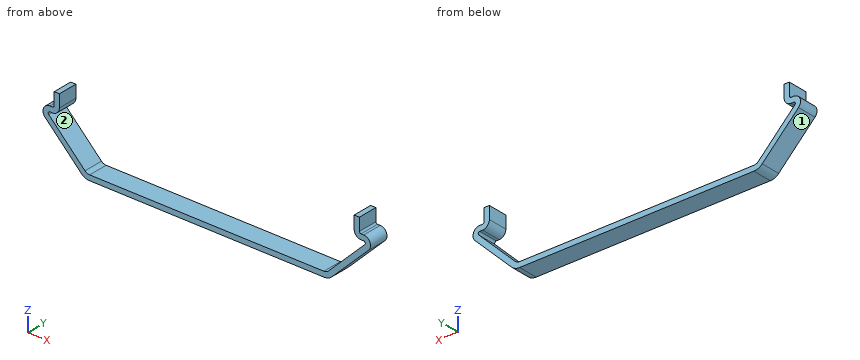
```python
from build123d import *

# Parameters (mm, degrees)
BOSS_EXTRUDE1_DEPTH = 1.5


with BuildPart() as part:
    # Sketch1 → Boss-Extrude1 (new, symmetric)
    with BuildSketch(Plane(origin=(0, 0, 0), x_dir=(1, 0, 0), z_dir=(0, 1, 0))):
        with BuildLine():
            Line((17.879536438, 11.70625), (-17.879536438, 11.70625))
            ThreePointArc((-17.879536438, 11.70625), (-18.26221987, 11.630129533), (-18.586643219, 11.413356781))
            Line((-18.586643219, 11.413356781), (-24.133026695, 5.866973305))
            ThreePointArc((-24.133026695, 5.866973305), (-24.187219883, 5.594525751), (-23.95625, 5.440196609))
            Line((-23.95625, 5.440196609), (-23.54375, 5.440196609))
            ThreePointArc((-23.54375, 5.440196609), (-22.805707297, 5.134489312), (-22.5, 4.396446609))
            Line((-22.5, 4.396446609), (-22.5, 2.5))
            Line((-22.5, 2.5), (-23.29375, 2.5))
            Line((-23.29375, 2.5), (-23.29375, 4.396446609))
            ThreePointArc((-23.29375, 4.396446609), (-23.366973305, 4.573223305), (-23.54375, 4.646446609))
            Line((-23.54375, 4.646446609), (-23.95625, 4.646446609))
            ThreePointArc((-23.95625, 4.646446609), (-24.920549262, 5.290770777), (-24.694292703, 6.428239312))
            Line((-24.694292703, 6.428239312), (-19.147909226, 11.974622789))
            ThreePointArc((-19.147909226, 11.974622789), (-18.565974844, 12.363458911), (-17.879536438, 12.5))
            Line((-17.879536438, 12.5), (17.879536438, 12.5))
            ThreePointArc((17.879536438, 12.5), (18.565974844, 12.363458911), (19.147909226, 11.974622789))
            Line((19.147909226, 11.974622789), (24.694292703, 6.428239312))
            ThreePointArc((24.694292703, 6.428239312), (24.920549262, 5.290770777), (23.95625, 4.646446609))
            Line((23.95625, 4.646446609), (23.54375, 4.646446609))
            ThreePointArc((23.54375, 4.646446609), (23.366973305, 4.573223305), (23.29375, 4.396446609))
            Line((23.29375, 4.396446609), (23.29375, 2.5))
            Line((23.29375, 2.5), (22.5, 2.5))
            Line((22.5, 2.5), (22.5, 4.396446609))
            ThreePointArc((22.5, 4.396446609), (22.805707297, 5.134489312), (23.54375, 5.440196609))
            Line((23.54375, 5.440196609), (23.95625, 5.440196609))
            ThreePointArc((23.95625, 5.440196609), (24.187219883, 5.594525751), (24.133026695, 5.866973305))
            Line((24.133026695, 5.866973305), (18.586643219, 11.413356781))
            ThreePointArc((18.586643219, 11.413356781), (18.26221987, 11.630129533), (17.879536438, 11.70625))
        make_face()
    extrude(amount=BOSS_EXTRUDE1_DEPTH, both=True)


solid = part.part
```
Geometry check sheet. Reference: the model listing, model coordinates, mm. Face numbers are marked on the shaded views. Give positions to 0.01 mm unless a question says otherwise; leave off trailing zeros. Order: outer loops, then holes, each group sorted by start corner. A loop starts at its lowest first (then second) coordinate and runs counter-clockwise, first axis right, second up.
1. Section check C-C, the plane x = -12.5. Enter the section's corners in (y, z).
2. Section check A-A, the plane z = -10.5. Enter the section's corners in (x, y), and give its area (3 significant figures).
3. Section check D-D, the plane x = 20.5. Enter the section's corners in (y, z).
4. Thickness scan on L1, parallel to X at y = -0.4, z = -3; L2, parallel to Z at x = -14, y = 0.25; L3, parallel to X at y = -0.1, z = -10. Record the ranges inside material, lowest first.
5. Release check for a two-part mould opening along Z. For the marked faces 1 and 2 record: pulls with the +Z half, pulls with the -Z half, needs draft (parallel to the pull), parting line crosses it, or undercut.
6. Section check B-B, the plane y = -0.75. Enter the section's corners in (x, z).
7. Gauge pin test, flat ends, axial feed: pin 1 Ø0.5 at (x, y) = (-23.5, 0.5) entering from +Z; pin 2 Ø1 at (x, y) = (-7.5, 1) entering from +Z; pin 3 Ø1.5 at (y, z) = (0, -3) entering from +X; pin 4 Ø0.9 at (y, z) = (0.5, -3.5) entering from -X. Record the tip position at first contact, or that the pin passes through.
Values follow:
1. outline: (-1.5, -12.5) - (1.5, -12.5) - (1.5, -11.71) - (-1.5, -11.71) - close
2. outline: (-20.62, -1.5) - (-19.5, -1.5) - (-19.5, 1.5) - (-20.62, 1.5) - close; (19.5, -1.5) - (20.62, -1.5) - (20.62, 1.5) - (19.5, 1.5) - close
2. area: 6.74 mm2
3. outline: (-1.5, -10.62) - (1.5, -10.62) - (1.5, -9.5) - (-1.5, -9.5) - close
4. L1: x = -23.29 to -22.5, 22.5 to 23.29
4. L2: z = -12.5 to -11.71
4. L3: x = -21.12 to -20, 20 to 21.12
5. face 1: pulls with the -Z half
5. face 2: undercut
6. outline: (-24.69, -6.43) - (-19.15, -11.97) arc R1.79 ccw to (-17.88, -12.5) - (17.88, -12.5) arc R1.79 ccw to (19.15, -11.97) - (24.69, -6.43) arc R1.04 ccw to (23.96, -4.65) - (23.54, -4.65) arc R0.25 cw to (23.29, -4.4) - (23.29, -2.5) - (22.5, -2.5) - (22.5, -4.4) arc R1.04 ccw to (23.54, -5.44) - (23.96, -5.44) arc R0.25 cw to (24.13, -5.87) - (18.59, -11.41) arc R1 cw to (17.88, -11.71) - (-17.88, -11.71) arc R1 cw to (-18.59, -11.41) - (-24.13, -5.87) arc R0.25 cw to (-23.96, -5.44) - (-23.54, -5.44) arc R1.04 ccw to (-22.5, -4.4) - (-22.5, -2.5) - (-23.29, -2.5) - (-23.29, -4.4) arc R0.25 cw to (-23.54, -4.65) - (-23.96, -4.65) arc R1.04 ccw to start
7. pin 1: stops at z = -2.5
7. pin 2: stops at z = -11.71
7. pin 3: stops at x = 23.29
7. pin 4: stops at x = -23.29
